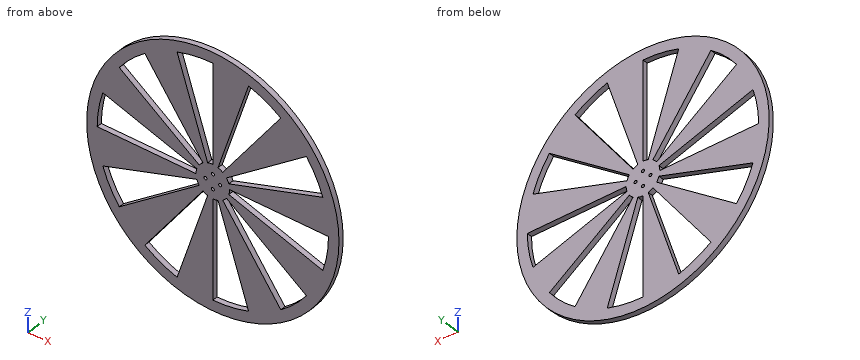
from build123d import *

# Parameters (mm, degrees)
SKETCH_1_R      = 120
SKETCH_1_R_2    = 1.45
EXTRUDE_1_DEPTH = 2.5


with BuildPart() as part:
    # 草图1 → 凸台-拉伸1 (new body, symmetric)
    with BuildSketch(Plane(origin=(0, 0, 0), x_dir=(1, 0, 0), z_dir=(0, 1, 0))):
        Circle(SKETCH_1_R)
        with Locations((7, 0)):
            Circle(SKETCH_1_R_2, mode=Mode.SUBTRACT)
        with Locations((0, 7)):
            Circle(SKETCH_1_R_2, mode=Mode.SUBTRACT)
        with Locations((-7, 0)):
            Circle(SKETCH_1_R_2, mode=Mode.SUBTRACT)
        with Locations((0, -7)):
            Circle(SKETCH_1_R_2, mode=Mode.SUBTRACT)
        with BuildLine():
            Line((16, 0), (110, 0))
            ThreePointArc((110, 0), (108.645717465, 17.207791154), (104.616216792, 33.991869381))
            Line((104.616216792, 33.991869381), (15.216904261, 4.94427191))
            ThreePointArc((15.216904261, 4.94427191), (15.80301345, 2.502951441), (16, 0))
        make_face(mode=Mode.SUBTRACT)
        with BuildLine():
            Line((9.404564037, 12.94427191), (64.656377752, 88.991869381))
            ThreePointArc((64.656377752, 88.991869381), (77.781745931, 77.781745931), (88.991869381, 64.656377752))
            Line((88.991869381, 64.656377752), (12.94427191, 9.404564037))
            ThreePointArc((12.94427191, 9.404564037), (11.313708499, 11.313708499), (9.404564037, 12.94427191))
        make_face(mode=Mode.SUBTRACT)
        with BuildLine():
            Line((0, 16), (0, 110))
            ThreePointArc((0, 110), (17.207791154, 108.645717465), (33.991869381, 104.616216792))
            Line((33.991869381, 104.616216792), (4.94427191, 15.216904261))
            ThreePointArc((4.94427191, 15.216904261), (2.502951441, 15.80301345), (0, 16))
        make_face(mode=Mode.SUBTRACT)
        with BuildLine():
            Line((-9.404564037, 12.94427191), (-64.656377752, 88.991869381))
            ThreePointArc((-64.656377752, 88.991869381), (-49.938954971, 98.010717661), (-33.991869381, 104.616216792))
            Line((-33.991869381, 104.616216792), (-4.94427191, 15.216904261))
            ThreePointArc((-4.94427191, 15.216904261), (-7.263847996, 14.256104387), (-9.404564037, 12.94427191))
        make_face(mode=Mode.SUBTRACT)
        with BuildLine():
            Line((-15.216904261, 4.94427191), (-104.616216792, 33.991869381))
            ThreePointArc((-104.616216792, 33.991869381), (-98.010717661, 49.938954971), (-88.991869381, 64.656377752))
            Line((-88.991869381, 64.656377752), (-12.94427191, 9.404564037))
            ThreePointArc((-12.94427191, 9.404564037), (-14.256104387, 7.263847996), (-15.216904261, 4.94427191))
        make_face(mode=Mode.SUBTRACT)
        with BuildLine():
            Line((-15.216904261, -4.94427191), (-104.616216792, -33.991869381))
            ThreePointArc((-104.616216792, -33.991869381), (-108.645717465, -17.207791154), (-110, 0))
            Line((-110, 0), (-16, 0))
            ThreePointArc((-16, 0), (-15.80301345, -2.502951441), (-15.216904261, -4.94427191))
        make_face(mode=Mode.SUBTRACT)
        with BuildLine():
            Line((-9.404564037, -12.94427191), (-64.656377752, -88.991869381))
            ThreePointArc((-64.656377752, -88.991869381), (-77.781745931, -77.781745931), (-88.991869381, -64.656377752))
            Line((-88.991869381, -64.656377752), (-12.94427191, -9.404564037))
            ThreePointArc((-12.94427191, -9.404564037), (-11.313708499, -11.313708499), (-9.404564037, -12.94427191))
        make_face(mode=Mode.SUBTRACT)
        with BuildLine():
            Line((0, -16), (0, -110))
            ThreePointArc((0, -110), (-17.207791154, -108.645717465), (-33.991869381, -104.616216792))
            Line((-33.991869381, -104.616216792), (-4.94427191, -15.216904261))
            ThreePointArc((-4.94427191, -15.216904261), (-2.502951441, -15.80301345), (0, -16))
        make_face(mode=Mode.SUBTRACT)
        with BuildLine():
            Line((9.404564037, -12.94427191), (64.656377752, -88.991869381))
            ThreePointArc((64.656377752, -88.991869381), (49.938954971, -98.010717661), (33.991869381, -104.616216792))
            Line((33.991869381, -104.616216792), (4.94427191, -15.216904261))
            ThreePointArc((4.94427191, -15.216904261), (7.263847996, -14.256104387), (9.404564037, -12.94427191))
        make_face(mode=Mode.SUBTRACT)
        with BuildLine():
            Line((15.216904261, -4.94427191), (104.616216792, -33.991869381))
            ThreePointArc((104.616216792, -33.991869381), (98.010717661, -49.938954971), (88.991869381, -64.656377752))
            Line((88.991869381, -64.656377752), (12.94427191, -9.404564037))
            ThreePointArc((12.94427191, -9.404564037), (14.256104387, -7.263847996), (15.216904261, -4.94427191))
        make_face(mode=Mode.SUBTRACT)
    extrude(amount=EXTRUDE_1_DEPTH, both=True)


solid = part.part
Part model, mm, in its own coordinate system. Give positions to 0.01 mm unless a question says otherwise; leave off trailing zeros. Loops run counter-clockwise (first coordinate to the right, second up) from the corner with the lowest first, then second, coordinate; pieces in that order, holes last. Notation, with made-up numbers: (12.25, 88.25) -> (48.25, 88.25) arc R12 cw to (48.25, 94.25) -> close; hole circle Ø10 at (-7.75, 81). An arc over 180 degrees is marked (long way). Write each question's results on one line, items separated by ' | '. Start each with the question number.
Q1. Band-saw the part on A-A on x = -22. List the corners of the cut face in (y, z).
Q2. Band-saw the part on C-C on x = 96. List the corners of the cut face in (y, z).
Q3. Pin check, flat tips, straight feed: P1, Ø1.5, axis at x = 65, y = -0.5, coming from the -Z side; P2, Ø2.5, axis at x = -81.5, y = -0.5, coming from the +Z side; P3, Ø2.5, axis at y = -0.5, z = 58.5, coming from the -X side. Stop position of each tip, or through.
Q4. Band-saw the part on D-D on z = 67.5. List the corners of the cut face in (x, y).
Q5. Wall check: L1, parallel to Z at x = 44.5, y = -1.6; L2, parallel to X at y = -0.4, z = 64; L3, parallel to X at y = 1.1, z = 73. Give the ranges that are in metal, low to high.
Q6. Band-saw the part on B-B on z = -101. List the corners of the cut face in (x, y), plus the area to 3 significant figures.
Results are:
1) outline: (-2.5, -117.97) -> (2.5, -117.97) -> (2.5, -67.71) -> (-2.5, -67.71) -> close; (-2.5, -30.28) -> (2.5, -30.28) -> (2.5, -15.98) -> (-2.5, -15.98) -> close; (-2.5, -7.15) -> (2.5, -7.15) -> (2.5, 0) -> (-2.5, 0) -> close; (-2.5, 7.15) -> (2.5, 7.15) -> (2.5, 15.98) -> (-2.5, 15.98) -> close; (-2.5, 30.28) -> (2.5, 30.28) -> (2.5, 67.71) -> (-2.5, 67.71) -> close; (-2.5, 107.78) -> (2.5, 107.78) -> (2.5, 117.97) -> (-2.5, 117.97) -> close
2) outline: (-2.5, -72) -> (2.5, -72) -> (2.5, -31.19) -> (-2.5, -31.19) -> close; (-2.5, 0) -> (2.5, 0) -> (2.5, 31.19) -> (-2.5, 31.19) -> close; (-2.5, 53.7) -> (2.5, 53.7) -> (2.5, 72) -> (-2.5, 72) -> close
3) P1: stops at z = -101.35 | P2: stops at z = 89.22 | P3: stops at x = -105.46
4) outline: (-99.22, -2.5) -> (-86.85, -2.5) -> (-86.85, 2.5) -> (-99.22, 2.5) -> close; (-49.04, -2.5) -> (-21.93, -2.5) -> (-21.93, 2.5) -> (-49.04, 2.5) -> close; (0, -2.5) -> (21.93, -2.5) -> (21.93, 2.5) -> (0, 2.5) -> close; (49.04, -2.5) -> (99.22, -2.5) -> (99.22, 2.5) -> (49.04, 2.5) -> close
5) L1: z = -111.44 to -61.25, -32.33 to -14.46, 0 to 14.46, 32.33 to 61.25, 100.6 to 111.44 | L2: x = -101.51 to -88.09, -46.5 to -20.79, 0 to 20.79, 46.5 to 88.09, 89.47 to 101.51 | L3: x = -95.24 to -82.29, -53.04 to -23.72, 0 to 23.72, 53.04 to 95.24
6) outline: (-64.8, -2.5) -> (-43.58, -2.5) -> (-43.58, 2.5) -> (-64.8, 2.5) -> close; (-32.82, -2.5) -> (0, -2.5) -> (0, 2.5) -> (-32.82, 2.5) -> close; (32.82, -2.5) -> (64.8, -2.5) -> (64.8, 2.5) -> (32.82, 2.5) -> close | area: 430 mm²
